Design review of the part built by this model. Coordinates are the model's own, in mm. A direction names the side the tool comes from. Coordinates: 2 decimals unless noted, no trailing zeros. Order: outer loops, then holes, each group sorted by start corner. A loop starts at its lowest first (then second) coordinate and runs counter-clockwise, first axis right, second up.
from build123d import *
from OCP.BRepFilletAPI import BRepFilletAPI_MakeChamfer

# Parameters (mm, degrees)
BOSS_EXTRUDE1_DEPTH             = 3.175
TAP_DRILL_FOR_M5X0_8_TAP1_D     = 4.2
BOSS_EXTRUDE2_DEPTH             = 3.175
TAP_DRILL_FOR_M5X0_8_TAP2_D     = 4.2
SKETCH11_R                      = 10
CUT_EXTRUDE3_DEPTH              = 3.175
TAP_DRILL_FOR_M4X0_7_TAP1_D     = 3.3
CUT_EXTRUDE5_DEPTH              = 3.175
CHAMFER1_SIZE                   = 2
CHAMFER1_SIZE2                  = 2.712078889
CHAMFER1_SIZE2_2                = 2.771226843
CUT_EXTRUDE6_START              = -9
CUT_EXTRUDE6_DEPTH              = 9
TAP_DRILL_FOR_M2X0_4_TAP1_D     = 1.6
TAP_DRILL_FOR_M2X0_4_TAP1_DEPTH = 3
TAP_DRILL_FOR_M2X0_4_TAP1_TIP   = 0.480688495


with BuildPart() as part:
    # Sketch1 → Boss-Extrude1 (new body)
    with BuildSketch(Plane.XY):
        with BuildLine():
            Line((-79, 10), (79, 10))
            ThreePointArc((79, 10), (89, 0), (79, -10))
            Line((79, -10), (-79, -10))
            ThreePointArc((-79, -10), (-89, 0), (-79, 10))
        make_face()
    extrude(amount=BOSS_EXTRUDE1_DEPTH)

    # Tap Drill for M5x0.8 Tap1 (through all)
    with Locations(Plane(origin=(0, 0, 0), x_dir=(-1, 0, 0), z_dir=(0, 0, -1))):
        with Locations((-79, 0), (79, 0)):
            Hole(TAP_DRILL_FOR_M5X0_8_TAP1_D / 2)

    # Sketch8 → Boss-Extrude2 (add)
    with BuildSketch(Plane(origin=(0, 0, 0), x_dir=(-1, 0, 0), z_dir=(0, 0, -1))):
        Polygon((29.25, 46.25), (7.25, 46.25), (-2, 10), (38, 10), align=None)
    extrude(amount=-BOSS_EXTRUDE2_DEPTH)

    # Tap Drill for M5x0.8 Tap2 (through all)
    with Locations(Plane(origin=(0, 0, 0), x_dir=(-1, 0, 0), z_dir=(0, 0, -1))):
        with Locations((7, 13), (29, 13)):
            Hole(TAP_DRILL_FOR_M5X0_8_TAP2_D / 2)

    # Sketch11 → Cut-Extrude3 (cut)
    with BuildSketch(Plane(origin=(0, 0, 0), x_dir=(-1, 0, 0), z_dir=(0, 0, -1))):
        with Locations((18, 32)):
            Circle(SKETCH11_R)
    extrude(amount=-CUT_EXTRUDE3_DEPTH, mode=Mode.SUBTRACT)

    # Tap Drill for M4x0.7 Tap1 (through all)
    with Locations(Plane(origin=(0, 0, 0), x_dir=(-1, 0, 0), z_dir=(0, 0, -1))):
        with Locations((0, 0), (-55, 0), (18, 13), (65, 0)):
            Hole(TAP_DRILL_FOR_M4X0_7_TAP1_D / 2)

    # Sketch17 → Cut-Extrude5 (cut)
    with BuildSketch(Plane(origin=(0, 0, 0), x_dir=(-1, 0, 0), z_dir=(0, 0, -1))):
        with BuildLine():
            Line((-73, 1.1), (-60, 1.1))
            ThreePointArc((-60, 1.1), (-58.9, 0), (-60, -1.1))
            Line((-60, -1.1), (-73, -1.1))
            ThreePointArc((-73, -1.1), (-74.1, 0), (-73, 1.1))
        make_face()
        with BuildLine():
            Line((-50, 1.1), (-5, 1.1))
            ThreePointArc((-5, 1.1), (-3.9, 0), (-5, -1.1))
            Line((-5, -1.1), (-50, -1.1))
            ThreePointArc((-50, -1.1), (-51.1, 0), (-50, 1.1))
        make_face()
        with BuildLine():
            Line((5, 1.1), (60, 1.1))
            ThreePointArc((60, 1.1), (61.1, 0), (60, -1.1))
            Line((60, -1.1), (5, -1.1))
            ThreePointArc((5, -1.1), (3.9, 0), (5, 1.1))
        make_face()
        with BuildLine():
            Line((70, 1.1), (73, 1.1))
            ThreePointArc((73, 1.1), (74.1, 0), (73, -1.1))
            Line((73, -1.1), (70, -1.1))
            ThreePointArc((70, -1.1), (68.9, 0), (70, 1.1))
        make_face()
    extrude(amount=-CUT_EXTRUDE5_DEPTH, mode=Mode.SUBTRACT)

    # Chamfer1: one chamfer whose edges measure the first distance from different faces: ONE call of the kernel's chamfer builder (chamfer() names one face for all edges)
    chamfer1_edges_1 = [part.edges().sort_by_distance(p)[0] for p in [
        (-38, 10, 1.5875),
    ]]
    chamfer1_side_1 = [part.faces().sort_by_distance(p)[0] for p in [
        (-33.625, 28.125, 1.5875),
    ]]
    chamfer1_edges_2 = [part.edges().sort_by_distance(p)[0] for p in [
        (2, 10, 1.5875),
    ]]
    chamfer1_side_2 = [part.faces().sort_by_distance(p)[0] for p in [
        (40.5, 10, 1.5875),
    ]]
    chamfer1 = BRepFilletAPI_MakeChamfer(part.part.solid().wrapped)
    for e in chamfer1_edges_1:
        chamfer1.Add(CHAMFER1_SIZE, CHAMFER1_SIZE2, e.wrapped, chamfer1_side_1[0].wrapped)  # the first distance lies on this face
    for e in chamfer1_edges_2:
        chamfer1.Add(CHAMFER1_SIZE, CHAMFER1_SIZE2_2, e.wrapped, chamfer1_side_2[0].wrapped)  # the first distance lies on this face
    add(Compound.cast(chamfer1.Shape()), mode=Mode.REPLACE)

    # Sketch18 → Cut-Extrude6 (cut)
    with BuildSketch(Plane.XY.offset(3.175).offset(CUT_EXTRUDE6_START)):
        with BuildLine():
            Line((4, 10), (5.5, 8.5))
            Line((5.5, 8.5), (73.732173124, 8.5))
            ThreePointArc((73.732173124, 8.5), (76.261387212, 9.617692031), (79, 10))
            Line((79, 10), (4, 10))
        make_face()
        with BuildLine():
            Line((-4, -10), (-79, -10))
            ThreePointArc((-79, -10), (-76.261387212, -9.617692031), (-73.732173124, -8.5))
            Line((-73.732173124, -8.5), (-5.5, -8.5))
            Line((-5.5, -8.5), (-4, -10))
        make_face()
    extrude(amount=CUT_EXTRUDE6_DEPTH, mode=Mode.SUBTRACT)

    # Tap Drill for M2x0.4 Tap1
    with Locations(Plane(origin=(0, 46.25, 0), x_dir=(1, 0, 0), z_dir=(0, 1, 0))):
        with Locations((-24.25, -1.5875), (-12.25, -1.5875)):
            Hole(TAP_DRILL_FOR_M2X0_4_TAP1_D / 2, depth=TAP_DRILL_FOR_M2X0_4_TAP1_DEPTH)
            with Locations((0, 0, -(TAP_DRILL_FOR_M2X0_4_TAP1_DEPTH + TAP_DRILL_FOR_M2X0_4_TAP1_TIP / 2))):  # 118° drill point
                Cone(0, TAP_DRILL_FOR_M2X0_4_TAP1_D / 2, TAP_DRILL_FOR_M2X0_4_TAP1_TIP, mode=Mode.SUBTRACT)


solid = part.part
1. Add section A-A (x = -65). Give the boundary of the cut face in (y, z) (3 decimals).
2. To check wall thickness, follow line 1 (Y direction, x = -29, z = 1.6); line 2 (Y direction, x = -18, z = 1.65); line 3 (Y direction, x = 61, z = 1.95). State the ranges of each line that lie inside material, in increasing order.
3. Mouldability with a two-part tool opening along Y and no side actions: class faces 1 (the flat face through (-6, 6, 3.175)), 2 (the cylindrical face through (-1.216, 1.115, 1.61)), 3 (the flat face through (-3.028, 29.703, 1.565)) as pulls with the +Y half, pulls with the -Y half, needs draft (parallel to the pull), parting line crosses it, or undercut.
4. For faces 4 (the flat face through (-33.448, 28.857, 1.565)), 5 (the flat face through (-40, -8.5, 2)), 6 (the flat face through (28, 1.1, 2)), list the 3-axis set-ups (+Z, -Z, +X, -X, +Y, -Y) from which the entire face can be reached by the end or side of a thin tool; tool diameter is ignored.
5. Add section C-C (x = -18). Give the boundary of the cut face in (y, z) (3 decimals), and give its area (3 significant figures).
6. Add section B-B (y = 35). Give the boundary of the cut face in (x, z) (3 decimals), and give its area (3 significant figures).
7. Insertion check: pin 1 (1 mm diameter, centred on x = -53, z = 1, fed in from +Y); pin 2 (1 mm diameter, centred on x = -12.25, z = 1.59, fed in from -Y); pin 3 (1.5 mm diameter, centred on y = 30.5, z = 2.5, fed in from -X). Each pin has a flat end and moves straight along its axis. Give the tip position at first contact, or say it passes through.
8. Add section D-D (y = 18.5). Give the boundary of the cut face in (x, z) (3 decimals).
Solution:
1. outline: (-8.5, 0) - (-1.65, 0) - (-1.65, 3.175) - (-8.5, 3.175) - close; (1.65, 0) - (10, 0) - (10, 3.175) - (1.65, 3.175) - close
2. line 1: y = -8.5 to -1.1, 1.1 to 10.9, 15.1 to 46.25
2. line 2: y = -8.5 to -1.1, 1.1 to 11.35, 14.65 to 22, 42 to 46.25
2. line 3: y = -10 to -1.1, 1.1 to 8.5
3. face 1: needs draft
3. face 2: undercut
3. face 3: pulls with the +Y half
4. face 4: +Z, -Z, -X, +Y
4. face 5: +Z, -Z, -Y
4. face 6: +Z, -Z
5. outline: (-8.5, 0) - (-1.1, 0) - (-1.1, 3.175) - (-8.5, 3.175) - close; (1.1, 0) - (11.35, 0) - (11.35, 3.175) - (1.1, 3.175) - close; (14.65, 0) - (22, 0) - (22, 3.175) - (14.65, 3.175) - close; (42, 0) - (46.25, 0) - (46.25, 3.175) - (42, 3.175) - close
5. area: 92.9 mm2
6. outline: (-31.966, 0) - (-27.539, 0) - (-27.539, 3.175) - (-31.966, 3.175) - close; (-8.461, 0) - (-4.379, 0) - (-4.379, 3.175) - (-8.461, 3.175) - close
6. area: 27.0 mm2
7. pin 1: stops at y = 10
7. pin 2: stops at y = -8.5
7. pin 3: stops at x = -33.23
8. outline: (-35.948, 0) - (-0.169, 0) - (-0.169, 3.175) - (-35.948, 3.175) - close
